```python
from build123d import *

# Parameters (mm, degrees)
EXTRUDE_1_DEPTH     = 15
SKETCH_2_R          = 2
CUT_EXTRUDE_1_DEPTH = 4
SKETCH_3_R          = 7.5
EXTRUDE_2_DEPTH     = 3
EXTRUDE_START       = -3
SKETCH_4_R          = 7.5
EXTRUDE_3_DEPTH     = 3
SKETCH_5_R          = 2
CUT_EXTRUDE_2_DEPTH = 11
EXTRUDE_4_DEPTH     = 4
SKETCH_6_R          = 0.75
CUT_EXTRUDE_3_DEPTH = 3
FILLET_1_R          = 2.5


with BuildPart() as part:
    # 草圖1 → 填料-伸長1 (new body)
    with BuildSketch(Plane.XY):
        Polygon((-24.89877099, 51.4), (-7.260334344, 29.1), (0, 29.1), (0, 26.1), (-6.196480976, 26.1), (-6.196480976, 21.1), (0, 21.1), (0, 18.1), (-7.5, 18.1), (-25, 0), (-51.696480976, 0), (-51.696480976, 4), (-47.696480976, 4), (-26.696480976, 4), (-9.196480976, 22.1), (-9.196480976, 25.1), (-16.981570729, 34.942567398), (-26.834917623, 47.4), (-41.746480973, 47.4), (-41.746480973, 51.4), align=None)
    extrude(amount=EXTRUDE_1_DEPTH)

    # 草圖2 → 除料-伸長1 (cut)
    with BuildSketch(Plane.XZ):
        with Locations((-46.696480976, 7.5)):
            Circle(SKETCH_2_R)
    extrude(amount=-CUT_EXTRUDE_1_DEPTH, mode=Mode.SUBTRACT)

    # 草圖3 → 填料-伸長2 (add)
    with BuildSketch(Plane.XZ.offset(-18.1)):
        with Locations((0, 7.5)):
            Circle(SKETCH_3_R)
    extrude(amount=-EXTRUDE_2_DEPTH)

    # 草圖4 → 填料-伸長3 (add)
    with BuildSketch(Plane(origin=(0, 29.1, 0), x_dir=(1, 0, 0), z_dir=(0, 1, 0)).offset(EXTRUDE_START)):
        with Locations((0, -7.5)):
            Circle(SKETCH_4_R)
    extrude(amount=EXTRUDE_3_DEPTH)

    # 草圖5 → 除料-伸長2 (cut)
    with BuildSketch(Plane(origin=(0, 29.1, 0), x_dir=(1, 0, 0), z_dir=(0, 1, 0))):
        with Locations(Location((0, -7.5, 0), (0, 0, 270))):
            Circle(SKETCH_5_R)
    extrude(amount=-CUT_EXTRUDE_2_DEPTH, mode=Mode.SUBTRACT)

    # 草圖7 → 填料-伸長4 (add)
    with BuildSketch(Plane(origin=(0, 51.4, 0), x_dir=(1, 0, 0), z_dir=(0, 1, 0))):
        with BuildLine():
            Line((-46.696480973, 2.5), (-46.696480973, -2.55))
            ThreePointArc((-46.696480973, -2.55), (-41.746480973, -7.5), (-46.696480973, -12.45))
            Line((-46.696480973, -12.45), (-46.696480973, -17.5))
            ThreePointArc((-46.696480973, -17.5), (-36.696480973, -7.5), (-46.696480973, 2.5))
        make_face()
    extrude(amount=-EXTRUDE_4_DEPTH)

    # 草圖6 → 除料-伸長3 (cut)
    with BuildSketch(Plane(origin=(0, 51.4, 0), x_dir=(1, 0, 0), z_dir=(0, 1, 0))):
        with Locations(Location((-39.196480973, -7.5, 0), (0, 0, 180))):
            Circle(SKETCH_6_R)
        with Locations(Location((-36.196480973, -7.5, 0), (0, 0, 180))):
            Circle(SKETCH_6_R)
        with Locations(Location((-33.196480973, -7.5, 0), (0, 0, 180))):
            Circle(SKETCH_6_R)
        with Locations(Location((-30.196480973, -7.5, 0), (0, 0, 180))):
            Circle(SKETCH_6_R)
    extrude(amount=-CUT_EXTRUDE_3_DEPTH, mode=Mode.SUBTRACT)

    # 圓角1
    fillet_1_edges = [part.edges().sort_by_distance(p)[0] for p in [
        (-51.696480976, 2, 0),
        (-51.696480976, 2, 15),
    ]]
    fillet(fillet_1_edges, radius=FILLET_1_R)


solid = part.part
```
The listing builds one solid part. Answer for the finished solid, in the listing's coordinates (mm). A direction names the side the tool comes from. Round coordinates to 2 decimals unless told otherwise and drop trailing zeros. Loops run counter-clockwise (first coordinate to the right, second up) from the corner with the lowest first, then second, coordinate; pieces in that order, holes last. Notation, with made-up numbers: (76, 67.25) -> (84, 67.25) arc R19 cw to (84, 81.25) -> close; hole circle Ø1 at (42, -38). An arc over 180 degrees is marked (long way). Use one line per item in the form item = value.
1. Flat-ended cylindrical pins translate along their axes: pin 1 Ø8 at (x, y) = (-44, 44) entering from -Z; pin 2 Ø1.2 at (y, z) = (49.5, 16) entering from -X; pin 3 Ø1.5 at (x, z) = (-10.5, 1) entering from +Y. Find the tip coordinate at first contact, or state that the pin passes through.
Answer key:
pin_1 = -2.48
pin_2 = -46.7
pin_3 = 34.14
2. A tool of negligible diameter and unlimited length cuts with its end or side. For faces 1 (the flat face through (-39, 48.4, 8)), 2 (the flat face through (-46.696, 49, 15)), 3 (the flat face through (-39, 4, 7)), 4 (the cylindrical face through (-41.748, 49.428, 7.391)), from which of +Z, -Z, +X, -X, +Y, -Y can it reach the whole face along a straight path? Write none if from no direction.
Answer key:
face_1 = +Y
face_2 = +Z, -Z, -X, +Y
face_3 = +Z, -Z, -X
face_4 = -X, +Y
3. The part is cut by section D-D on y = 7.5. Determine the outline of the cut face in (x, z).
Answer key:
outline = (-23.31, 0) -> (-17.75, 0) -> (-17.75, 15) -> (-23.31, 15) -> close
4. The part is cut by section A-A on x = -28. Determine the outline of the cut face in (y, z), and give its area (3 significant figures).
Answer key:
outline = (0, 0) -> (4, 0) -> (4, 15) -> (0, 15) -> close; (47.4, 0) -> (51.4, 0) -> (51.4, 15) -> (47.4, 15) -> close
area = 120 mm²
5. For a pull along Z with two mould halves and no side action, classify faces 5 (the flat face through (-2.5, 21.1, 7.6)), 6 (the flat face through (-36, 48.4, 8)), 7 (the cylindrical face through (-43.114, 49.428, -1.836)), 8 (the cylindrical face through (0.088, 19.621, 5.502)) as released by +Z, released by -Z, zero draft, split by the parting line, or undercut.
Answer key:
face_5 = zero draft
face_6 = undercut
face_7 = released by -Z
face_8 = undercut
6. The part is cut by section C-C on z = 1.75. Determine the outline of the cut face in (x, y), and give its area (3 significant figures).
Answer key:
outline = (-51.58, 0) -> (-25, 0) -> (-7.5, 18.1) -> (4.82, 18.1) -> (4.82, 21.1) -> (-6.2, 21.1) -> (-6.2, 26.1) -> (4.82, 26.1) -> (4.82, 29.1) -> (-7.26, 29.1) -> (-24.9, 51.4) -> (-46.7, 51.4) -> (-46.7, 47.4) -> (-26.83, 47.4) -> (-9.2, 25.1) -> (-9.2, 22.1) -> (-26.7, 4) -> (-51.58, 4) -> close
area = 492 mm²
7. Find the intervals of material crossed by probe 1 along Y at (x, z) = (-35, 5.75); probe 2 along X at (y, z) = (28.4, 7.5); probe 3 along X at (y, z) = (25, 9.25), in increasing order. Write a range as [from, to].
Answer key:
probe_1 = [0, 4], [47.4, 51.4]
probe_2 = [-11.81, -2], [2, 7.5]
probe_3 = [-9.2, -6.2]
8. The part is cut by section B-B on z = 7.5. Give the number of separate pieces and of enclosed holes in the cut face, and give its area (3 significant figures).
Answer key:
separate_pieces = 4
enclosed_holes = 0
area = 431 mm²
